```python
from build123d import *

# Parameters (mm, degrees)
SKETCH1_W           = 8
SKETCH1_H           = 50
BOSS_EXTRUDE1_DEPTH = 50
CUT_EXTRUDE1_DEPTH  = 72.161787499
FILLET1_R           = 3


with BuildPart() as part:
    # Sketch1 → Boss-Extrude1 (new body)
    with BuildSketch(Plane.XY):
        with Locations((4, 25)):
            Rectangle(SKETCH1_W, SKETCH1_H)
    extrude(amount=BOSS_EXTRUDE1_DEPTH)

    # Sketch2 → Cut-Extrude1 (cut, through all)
    with BuildSketch(Plane.ZY):
        Polygon((9, 0), (50, 45), (50, 0), align=None)
        with BuildLine():
            Line((34.919366889, 40.326510004), (27.939173676, 32.665322332))
            ThreePointArc((27.939173676, 32.665322332), (27.661132031, 32.43550968), (27.330075217, 32.292253277))
            Line((27.330075217, 32.292253277), (9.264065377, 27.346080088))
            ThreePointArc((9.264065377, 27.346080088), (8.393396908, 27.515580036), (8, 28.310584871))
            Line((8, 28.310584871), (8, 41))
            ThreePointArc((8, 41), (8.292893219, 41.707106781), (9, 42))
            Line((9, 42), (34.180170551, 42))
            ThreePointArc((34.180170551, 42), (35.094908218, 41.404048267), (34.919366889, 40.326510004))
        make_face()
        with BuildLine():
            Line((19.677865993, 23.598033411), (10.229578577, 13.227961857))
            ThreePointArc((10.229578577, 13.227961857), (8.819028368, 12.895892811), (8, 14.091348489))
            Line((8, 14.091348489), (8, 21.874636004))
            ThreePointArc((8, 21.874636004), (8.262795417, 22.65227636), (8.943438089, 23.111091691))
            Line((8.943438089, 23.111091691), (18.391725505, 25.697875729))
            ThreePointArc((18.391725505, 25.697875729), (19.823445803, 25.130997871), (19.677865993, 23.598033411))
        make_face()
    extrude(amount=-CUT_EXTRUDE1_DEPTH, mode=Mode.SUBTRACT)

    # Fillet1
    fillet1_edges = [part.edges().sort_by_distance(p)[0] for p in [
        (4, 0, 9),
        (4, 45, 50),
    ]]
    fillet(fillet1_edges, radius=FILLET1_R)


solid = part.part
```
Can you work these out from the model? Positions are in its coordinate system, mm. A direction names the side the tool comes from. Give positions to 0.01 mm unless a question says otherwise; leave off trailing zeros. Loops run counter-clockwise (first coordinate to the right, second up) from the corner with the lowest first, then second, coordinate; pieces in that order, holes last. Notation, with made-up numbers: M 19.25,-7.75 L 54.25,-7.75 A28 cw 54.25,25.25 Z; hole C 33,40 d3. An arc over 180 degrees is marked long. Use one line per item in the form item = value. Start each with the question number.
(1) On a 3-axis mill with a long thin cutter (end or side, diameter ignored), from which of +Z, -Z, +X, -X, +Y, -Y can I reach the whole of each face in a straight line? I mean faces 1 (the cylindrical face through (3.94, 27.51, 8.4)), 2 (the flat face through (8, 25, 14)). Say none if no direction works.
(2) I want a section at B-B, the plane x = 1.5. Write out the boundary of the cut face in (y, z), and give its area (3 significant figures).
(3) Thinking about a two-plate mould opening in Y: for faces 3 (the flat face through (4, 48, 50)), 4 (the flat face through (4, 0, 4)), 5 (the cylindrical face through (3.94, 25.15, 19.81)), 6 (the flat face through (3.944, 18.486, 15.02)), which applies, released by +Y, released by -Y, zero draft, split by the parting line, or undercut?
(4) I'm going to push flat-ended pins straight in: P1, Ø4, axis at x = 4, y = 17.5, coming from the +Z side; P2, Ø2.5, axis at x = 2.5, y = 37.5, coming from the +Z side; P3, Ø4, axis at x = 4.5, z = 23, coming from the -Y side; P4, Ø3, axis at y = 9, z = 20, coming from the +X side. Where does each tip first touch, or does it pass through?
(5) I want a section at A-A, the plane y = 34. Write out the boundary of the cut face in (x, z), and give its area (3 significant figures).
(6) Please list where these lines run through material, in increasing order: line 1 (Y direction, x = 3, z = 13); line 2 (Y direction, x = 1.75, z = 9.5); line 3 (Z direction, x = 6.75, y = 34.5).
(7) I want a section at D-D, the plane z = 12. Write out the boundary of the cut face in (x, y), and give its area (3 significant figures).
(8) I want a section at C-C, the plane z = 22. Write out the boundary of the cut face in (x, y).
Worked out:
q1.face_1 = +X, -X
q1.face_2 = +Z, -Z, +X, +Y, -Y
q2.outline = M 0,0 L 50,0 L 50,50 L 46.16,50 A3 ccw 44.14,49.22 L 0.98,9.89 A3 ccw 0,7.67 Z; hole M 13.23,10.23 A1.28 ccw 14.09,8 L 21.87,8 A1.28 ccw 23.11,8.94 L 25.7,18.39 A1.28 ccw 23.6,19.68 Z; hole M 27.35,9.26 A1 ccw 28.31,8 L 41,8 A1 ccw 42,9 L 42,34.18 A1 ccw 40.33,34.92 L 32.67,27.94 A1.28 ccw 32.29,27.33 Z
q2.area = 1,210 mm²
q3.face_3 = zero draft
q3.face_4 = released by -Y
q3.face_5 = undercut
q3.face_6 = undercut
q4.P1 = 26.77
q4.P2 = 44.31
q4.P3 = 13.17
q4.P4 = through
q5.outline = M 0,0 L 8,0 L 8,8 L 0,8 Z; M 0,29.16 L 8,29.16 L 8,39.98 L 0,39.98 Z
q5.area = 151 mm²
q6.line_1 = 4.39 to 16.27, 24.22 to 28.37, 42 to 50
q6.line_2 = 0.62 to 12.83, 23.26 to 27.41, 42 to 50
q6.line_3 = 0 to 8, 29.61 to 40.43
q7.outline = M 0,3.29 L 8,3.29 L 8,15.17 L 0,15.17 Z; M 0,23.95 L 8,23.95 L 8,28.1 L 0,28.1 Z; M 0,42 L 8,42 L 8,50 L 0,50 Z
q7.area = 192 mm²
q8.outline = M 0,14.27 L 8,14.27 L 8,30.83 L 0,30.83 Z; M 0,42 L 8,42 L 8,50 L 0,50 Z
